from build123d import *

# Parameters (mm, degrees)
SM_BASE_FLANGE_1_DEPTH = 393.5
SKETCH_3_R             = 3
CUT_EXTRUDE_1_DEPTH    = 396.780557885


# Sheet-metal steps are written as plain solids
with BuildPart() as part:
    # Sketch 1 → Базовая кромка1 (new, symmetric)
    with BuildSketch(Plane(origin=(0, 0, 0), x_dir=(0, 0, -1), z_dir=(1, 0, 0))):
        with BuildLine():
            Line((0, 0), (0, 22))
            ThreePointArc((0, 22), (2.343145751, 27.656854249), (8, 30))
            Line((8, 30), (30, 30))
            Line((30, 30), (30, 27))
            Line((30, 27), (8, 27))
            ThreePointArc((8, 27), (4.464466094, 25.535533906), (3, 22))
            Line((3, 22), (3, 0))
            Line((3, 0), (0, 0))
        make_face()
    extrude(amount=SM_BASE_FLANGE_1_DEPTH, both=True)

    # Эскиз3 → Вырез-Вытянуть1 (cut, through all)
    with BuildSketch(Plane.XY):
        with Locations((300, 10)):
            Circle(SKETCH_3_R)
        with Locations((-300, 10)):
            Circle(SKETCH_3_R)
    extrude(amount=-CUT_EXTRUDE_1_DEPTH, mode=Mode.SUBTRACT)


solid = part.part
Geometry check sheet. Reference: the model listing, model coordinates, mm. A direction names the side the tool comes from. Give positions to 0.01 mm unless a question says otherwise; leave off trailing zeros. Order: outer loops, then holes, each group sorted by start corner. A loop starts at its lowest first (then second) coordinate and runs counter-clockwise, first axis right, second up. Notation, with made-up numbers: (25, -32) - (70, -32) arc R27 cw to (70, 1) - close; hole circle Ø5 at (18.25, 62.5). An arc over 180 degrees is marked (long way). Use one line per item in the form item = value.
1) Sectioned sample at B-B (z = -20.25). Record the boundary of the cut face in (x, y), and give its area (3 significant figures).
Working result:
outline = (-393.5, 27) - (393.5, 27) - (393.5, 30) - (-393.5, 30) - close
area = 2,360 mm^2
2) Depth check by flat-ended pin: pin 1 Ø8 at (x, z) = (137.5, -16) entering from -Y; pin 2 Ø6.5 at (x, y) = (7, 13.5) entering from -Z. Enter the tip coordinate at first touch or a pass-through.
Working result:
pin_1 = 27
pin_2 = -3
3) Sectioned sample at A-A (x = -82). Record the boundary of the cut face in (y, z), and give its area (3 significant figures).
Working result:
outline = (0, -3) - (22, -3) arc R5 cw to (27, -8) - (27, -30) - (30, -30) - (30, -8) arc R8 ccw to (22, 0) - (0, 0) - close
area = 163 mm^2
4) Material ranges on probe 1 along Z at (x, y) = (-21.5, 6); probe 2 along Y at (x, z) = (207.5, -19.5); probe 3 along Y at (x, z) = (300, -1.8), recorded low to high. Write a range as from..to.
Working result:
probe_1 = -3..0
probe_2 = 27..30
probe_3 = 0..7, 13..27.06
5) Access from +Z, -Z, +X, -X, +Y, -Y to the whole of each face (thin tool, end or side, straight path). Record for faces 1 (the face through (-393.5, 27.3, -10.6)), 2 (the face through (6, 11, -3)).
Working result:
face_1 = +Z, -Z, -X, +Y, -Y
face_2 = -Z, +X, -X, -Y
